Part model, mm, in its own coordinate system. Give positions to 0.01 mm unless a question says otherwise; leave off trailing zeros. Loops run counter-clockwise (first coordinate to the right, second up) from the corner with the lowest first, then second, coordinate; pieces in that order, holes last. Notation, with made-up numbers: (72.5, 73) -> (129.5, 73) arc R27 ccw to (129.5, 107) -> close; hole circle Ø10 at (36, 79.25). An arc over 180 degrees is marked (long way). One line per question, with ' | ' between items.
Autodesk Inventor part; units mm, degrees
ref_plane "YZ Plane" through (0, 0, 0) normal (1, 0, 0) x (0, 1, 0)
ref_plane "XZ Plane" through (0, 0, 0) normal (0, 1, 0) x (-1, 0, 0)
ref_plane "XY Plane" through (0, 0, 0) normal (0, 0, 1) x (1, 0, 0)
sketch "Sketch1" plane through (0, 0, 0) normal (0, 0, 1) x (1, 0, 0)
  circle A0 centre (25.0838, -31.7051) radius 2.5
  circle A1 centre (43.012, -13.2629) radius 2.5
  circle A2 centre (44.8914, 13.7567) radius 2.5
  circle A3 centre (28.0838, 36.7109) radius 2.5
  circle A4 centre (-0.8935, 43.7288) radius 2.5
  circle A5 centre (-29.5533, 30.4373) radius 2.5
  circle A6 centre (-43.6662, -0.0951) radius 2.5
  circle A7 centre (-47.6662, -52.5951) radius 2.5
  circle A8 centre (-10.6662, -52.5951) radius 2.5
  circle A9 centre (6.8338, -0.0951) radius 4
  line L0 (-3.1662, -60.0951) -> (-3.1662, -40.8213)
  spline S0 degree 4 poles (-3.1662, -40.8213) (8.3823, -44.3792) (29.645, -43.1708) (54.7055, -22.2338) (56.6662, 18.5311) (25.1104, 60.0951) (-26.25, 55.8136) (-50.0319, 24.6801) (-51.1662, -0.0951) knots -0.895347 -0.895347 -0.895347 -0.895347 -0.895347 -0.704438 -0.582312 -0.457579 -0.330099 0 0 0 0 0
  line L1 (-51.1662, -0.0951) -> (-56.6662, -60.0951)
  line L2 (-56.6662, -60.0951) -> (-3.1662, -60.0951)
  circle A10 centre (6.8338, -0.0951) radius 11.2
  line L3 (-3.1662, -40.8213) -> (-29.9162, -34.2051) construction
  line L4 (-29.9162, -34.2051) -> (-46.1662, -23.5051) construction
  line L5 (-46.1662, -23.5051) -> (-51.1662, -0.0951) construction
  spline S1 degree 3 poles (-3.1662, -40.8213) (-29.9162, -34.2051) (-46.1662, -23.5051) (-51.1662, -0.0951) knots 1 1 1 1 2 2 2 2
  point P0 (0, 0)
  dimension "d0" = 22.4
extrude "Extrusion1" add sketch "Sketch1" along normal blind 2 contours S1 S0
sketch "Sketch2" plane through (0, 0, 2) normal (0, 0, 1) x (1, 0, 0)
  point P0 (0, 0)
sketch "Sketch3" plane through (0, 0, 2) normal (0, 0, 1) x (1, 0, 0)
  circle A0 centre (6.8338, -0.0951) radius 11.2
  circle A1 centre (6.8338, -0.0951) radius 14.2
  point P0 (0, 0)
  dimension "d3" = 3
extrude "Extrusion2" add sketch "Sketch3" along normal blind 8
sketch "Sketch4" plane through (0, 0, 2) normal (0, 0, 1) x (1, 0, 0)
  spline S0 degree 4 poles (-3.1662, -40.8213) (-27.2692, -5.9695) (-29.39, 39.4497) (49.0675, 34.0752) (52.786, 13.0688) knots 0 0 0 0 0 1 1 1 1 1
  circle A0 centre (6.8338, -0.0951) radius 14.2
  spline S1 degree 4 poles (-3.1662, -40.8213) (8.3823, -44.3792) (29.645, -43.1708) (54.7055, -22.2338) (56.6662, 18.5311) (25.1104, 60.0951) (-26.25, 55.8136) (-50.0319, 24.6801) (-51.1662, -0.0951) knots 0 0 0 0 0 0.213223 0.349624 0.488937 0.631318 1 1 1 1 1
  spline S2 degree 3 poles (-51.1662, -0.0951) (-46.1662, -23.5051) (-29.9162, -34.2051) (-3.1662, -40.8213) knots 0 0 0 0 1 1 1 1
  circle A1 centre (-43.6662, -0.0951) radius 2.5
  circle A2 centre (-29.5533, 30.4373) radius 2.5
  circle A3 centre (-0.8935, 43.7288) radius 2.5
  circle A4 centre (28.0838, 36.7109) radius 2.5
  circle A5 centre (44.8914, 13.7567) radius 2.5
  circle A6 centre (43.012, -13.2629) radius 2.5
  circle A7 centre (25.0838, -31.7051) radius 2.5
  point P0 (0, 0)
  point P1 (-15.7615, 0.0764)
  point P2 (0.4982, 21.7961)
  point P3 (35.8374, 25.3182)
  point P4 (52.5916, 13.9044)
extrude "Extrusion3" cut sketch "Sketch4" against normal blind 8 contours S2 S1 S0
properties part number "Estructura"
1) Drill centre lines: line 1 (Z direction, x = -5.5, y = 7); line 2 (Y direction, x = 41, z = 1.75); line 3 (X direction, y = -8, z = 9). Where is each one in solid material? Low to high.
Found:
line 1: 0 to 2 | line 2: -29.31 to -14.75, -11.78 to 23.73 | line 3: -4.96 to -1.1, 14.77 to 18.63
2) Pull direction Y, two halves, no side cores. Call faces 1 (the cylindrical face through (47.201, 14.714, 0.986)), 2 (the cylindrical face through (-4.43, 8.55, 5.94)), 3 (the flat face through (22, -2, 2)): pulls with the +Y half, pulls with the -Y half, needs draft (parallel to the pull), parting line crosses it, or undercut.
Found:
face 1: undercut | face 2: parting line crosses it | face 3: needs draft
3) Pin check, flat tips, straight feed: P1, Ø10, axis at x = 46.5, y = 3, coming from the -Z side; P2, Ø4.5, axis at x = 25.08, y = -31.71, coming from the +Z side; P3, Ø2, axis at y = -6, z = 6, coming from the -X side; P4, Ø2, axis at y = -3, z = 1.5, coming from the -X side. Stop position of each tip, or through.
Found:
P1: z = 0 | P2: through | P3: x = -6.49 | P4: x = -16.17
4) Saw through at A-A (z = 6). Give the cut face in (x, y).
Found:
outline: circle Ø28.4 at (6.83, -0.1); hole circle Ø22.4 at (6.83, -0.1)
